Autodesk Inventor part; units mm, degrees
ref_plane "YZ Plane" through (0, 0, 0) normal (1, 0, 0) x (0, 1, 0)
ref_plane "XZ Plane" through (0, 0, 0) normal (0, 1, 0) x (-1, 0, 0)
ref_plane "XY Plane" through (0, 0, 0) normal (0, 0, 1) x (1, 0, 0)
sketch "Sketch1" plane through (0, 0, 0) normal (0, 0, 1) x (1, 0, 0)
  line L0 (0, 0) -> (0.5, 0)
  line L1 (1, 1) -> (1, 4)
  line L2 (1, 4) -> (0, 4)
  line L3 (0, 4) -> (0, 0)
  arc A0 (0.5, 0) -> (1, 0.5) centre (0.5, 0.5) ccw
  line L4 (1, 0.5) -> (0.85, 0.5)
  line L5 (0.85, 0.5) -> (0.85, 1)
  line L6 (0.85, 1) -> (1, 1)
  point P0 (1, 0)
  dimension "d0" = 1
  dimension "d1" = 4
  dimension "d2" = 0.5
  dimension "d6" = 0.15
  dimension "d7" = 0.5
revolve "Revolution1" add sketch "Sketch1" angle 360 about axis through (0, 4, 0) along (0, -1, 0)
thread "Thread1"
sketch "Sketch2" plane through (0, 4, 0) normal (0, 1, 0) x (1, 0, 0)
  circle A0 centre (0, 0) radius 0.5
  circle A1 centre (0, 0) radius 1.75 construction
  line L0 (-1.5102, -0.8843) -> (-1.5209, 0.8657)
  line L1 (-1.5209, 0.8657) -> (-0.0107, 1.75)
  line L2 (-0.0107, 1.75) -> (1.5102, 0.8843)
  line L3 (1.5102, 0.8843) -> (1.5209, -0.8657)
  line L4 (1.5209, -0.8657) -> (0.0107, -1.75)
  line L5 (0.0107, -1.75) -> (-1.5102, -0.8843)
  dimension "d8" = 3.5
extrude "Extrusion1" add sketch "Sketch2" along normal blind 1
extrude "Extrusion2" add sketch "Sketch2" along normal blind 4 contours A0
fillet "Fillet1" radius 0.25 1 edges at (-0.5, 8, 0)
properties part number "temperature sensor"
For this review, take the finished solid that the model builds, in its own axes (mm). A direction names the side the tool comes from. Give positions to 0.01 mm unless a question says otherwise; leave off trailing zeros. Write each loop counter-clockwise with the first axis right and the second up, starting at its lowest first coordinate (ties: lowest second). Pieces come first, ordered by that corner, then holes. Notation, with made-up numbers: (87.5, -20) -> (142.5, -20) arc R18 ccw to (142.5, -13) -> close; hole circle Ø9 at (65.25, 54.25). An arc over 180 degrees is marked (long way). Use CSV: the item, a comma, the result in double quotes.
Q1. To check wall thickness, follow probe 1 along Y at (x, z) = (1.15, 0.85); probe 2 along Z at (x, y) = (-0.5, 2.75); probe 3 along Y at (x, z) = (0.5, 0.4). State the ranges of each line that lie inside material, in increasing order. Write a range as [from, to].
Conclusion:
probe 1,"[4, 5]"
probe 2,"[-0.87, 0.87]"
probe 3,"[0.02, 5]"
Q2. Take a section at B-B, the plane z = 1.2. Write out the cut boundary in (x, y).
Conclusion:
outline,"(-0.96, 4) -> (0.95, 4) -> (0.95, 5) -> (-0.96, 5) -> close"
Q3. Take a section at C-C, the plane x = -1.2. Write out the cut boundary in (y, z), then the cut area to 3 significant figures.
Conclusion:
outline,"(4, -1.05) -> (5, -1.05) -> (5, 1.06) -> (4, 1.06) -> close"
area,"2.11 mm2"
Q4. Take a section at D-D, the plane y = 5.75. Write out the cut boundary in (x, z), then the cut area to 3 significant figures.
Conclusion:
outline,"circle Ø1 at (0, 0)"
area,"0.785 mm2"
Q5. Mouldability with a two-part tool opening along Y and no side actions: class faces 1 (the face through (-0.18, 0.75, 0.83)), 2 (the face through (0, 3, 1)), 3 (the face through (0, 0, 0)), 4 (the face through (-1, 5, 0)) as pulls with the +Y half, pulls with the -Y half, needs draft (parallel to the pull), parting line crosses it, or undercut.
Conclusion:
face 1,"undercut"
face 2,"needs draft"
face 3,"pulls with the -Y half"
face 4,"pulls with the +Y half"
Q6. Tool access review of faces 5 (the face through (-0.78, 4.49, -1.3)), 6 (the face through (-1, 4, 1)), 7 (the face through (-0.108, 6.356, -0.488)): name each direction out of +Z, -Z, +X, -X, +Y, -Y from which nothing blocks a thin tool from reaching the whole face with its end or side.
Conclusion:
face 5,"-Z, -X, +Y, -Y"
face 6,"-Y"
face 7,"+Y"
Q7. Take a section at A-A, the plane y = 4.5. Write out the cut boundary in (x, z), then the cut area to 3 significant figures.
Conclusion:
outline,"(-1.52, -0.87) -> (-0.01, -1.75) -> (1.51, -0.88) -> (1.52, 0.87) -> (0.01, 1.75) -> (-1.51, 0.88) -> close"
area,"7.96 mm2"
Q8. For P1, Ø0.9, axis at x = 0.5, z = -0.5, coming from the -Y side, flat-tipped, find the tip position at first contact; note if it passes through.
Conclusion:
P1,"y = 0"
